Design review of the part built by this model. Coordinates are the model's own, in mm. Face numbers are marked on the shaded views. Coordinates: 2 decimals unless noted, no trailing zeros. Loops run counter-clockwise (first coordinate to the right, second up) from the corner with the lowest first, then second, coordinate; pieces in that order, holes last.
Q1. Add section B-B on z = 0. Give the boundary of the cut face in (x, y), and give its area (3 significant figures).
Q2. Wall thickness on probe 1 along X at (y, z) = (5.6, 0); probe 2 along X at (y, z) = (3.1, 0); probe 3 along Z at (x, y) = (-4, 1.75): over which ranges is each line inside the solid? List them lowest first.
Q3. Add section C-C on y = 5.75. Give the boundary of the cut face in (x, z).
Q4. Draft analysis for pull direction X (two halves, no side actions). For the marked faces 1, 2 and 3, state which applies: released by +X, released by -X, zero draft, split by the parting line, or undercut.
Q5. Add section D-D on y = 1. Give the boundary of the cut face in (x, z).
Q6. Add section A-A on x = 0. Give the boundary of the cut face in (y, z), and give its area (3 significant figures).
Q7. For P1, Ø3, axis at x = 0, z = 7.5, coming from the +Y side; P2, Ø3, axis at y = 3.5, z = 4, coming from the -X side; P3, Ø3, axis at x = 4, y = 2.5, coming from the -Z side, all flat-tipped, find the tip position at first contact; note any pin that passes through.
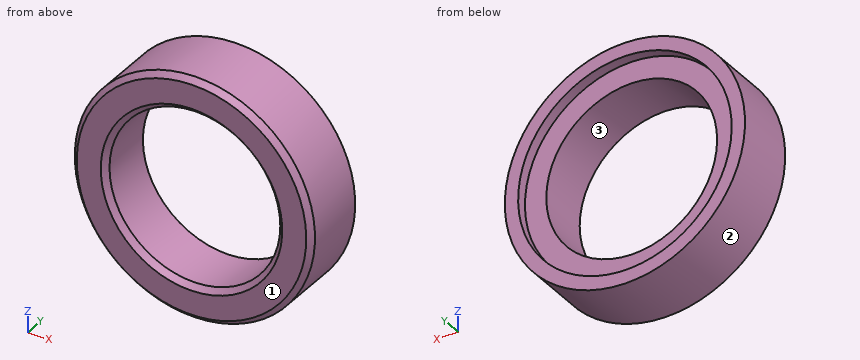
```python
from build123d import *

# Parameters (mm, degrees)
SKETCH1_R           = 11.25
SKETCH1_R_2         = 8
BOSS_EXTRUDE1_DEPTH = 6.4
SKETCH2_R           = 10
CUT_EXTRUDE1_DEPTH  = 1
CHAMFER1_SIZE       = 0.5


with BuildPart() as part:
    # Sketch1 → Boss-Extrude1 (new body)
    with BuildSketch(Plane(origin=(0, 0, 0), x_dir=(1, 0, 0), z_dir=(0, 1, 0))):
        with Locations(Location((0, 0, 0), (0, 0, 270))):
            Circle(SKETCH1_R)
        with Locations(Location((0, 0, 0), (0, 0, 270))):
            Circle(SKETCH1_R_2, mode=Mode.SUBTRACT)
    extrude(amount=BOSS_EXTRUDE1_DEPTH)

    # Sketch2 → Cut-Extrude1 (cut)
    with BuildSketch(Plane(origin=(0, 6.4, 0), x_dir=(1, 0, 0), z_dir=(0, 1, 0))):
        with Locations(Location((0, 0, 0), (0, 0, 270))):
            Circle(SKETCH2_R)
    extrude(amount=-CUT_EXTRUDE1_DEPTH, mode=Mode.SUBTRACT)

    # Chamfer1
    chamfer1_edges = [part.edges().sort_by_distance(p)[0] for p in [
        (0, 0, -11.25),
        (0, 0, -8),
    ]]
    chamfer(chamfer1_edges, length=CHAMFER1_SIZE)


solid = part.part
```
Entries:
1. outline: (-11.25, 0.5) - (-10.75, 0) - (-8.5, 0) - (-8, 0.5) - (-8, 5.4) - (-10, 5.4) - (-10, 6.4) - (-11.25, 6.4) - close; (8, 0.5) - (8.5, 0) - (10.75, 0) - (11.25, 0.5) - (11.25, 6.4) - (10, 6.4) - (10, 5.4) - (8, 5.4) - close
1. area: 37.1 mm2
2. probe 1: x = -11.25 to -10, 10 to 11.25
2. probe 2: x = -11.25 to -8, 8 to 11.25
2. probe 3: z = -10.51 to -6.93, 6.93 to 10.51
3. outline: circle Ø22.5 at (0, 0); hole circle Ø20 at (0, 0)
4. face 1: zero draft
4. face 2: split by the parting line
4. face 3: undercut
5. outline: circle Ø22.5 at (0, 0); hole circle Ø16 at (0, 0)
6. outline: (0, -10.75) - (0.5, -11.25) - (6.4, -11.25) - (6.4, -10) - (5.4, -10) - (5.4, -8) - (0.5, -8) - (0, -8.5) - close; (0, 8.5) - (0.5, 8) - (5.4, 8) - (5.4, 10) - (6.4, 10) - (6.4, 11.25) - (0.5, 11.25) - (0, 10.75) - close
6. area: 37.1 mm2
7. P1: stops at y = 5.4
7. P2: stops at x = -10.97
7. P3: stops at z = -10.97
